Source: CAD feature listing. Evaluate the final solid. Frame: model axes, mm. Give positions to 0.01 mm unless a question says otherwise; leave off trailing zeros. Order: outer loops, then holes, each group sorted by start corner. A loop starts at its lowest first (then second) coordinate and runs counter-clockwise, first axis right, second up.
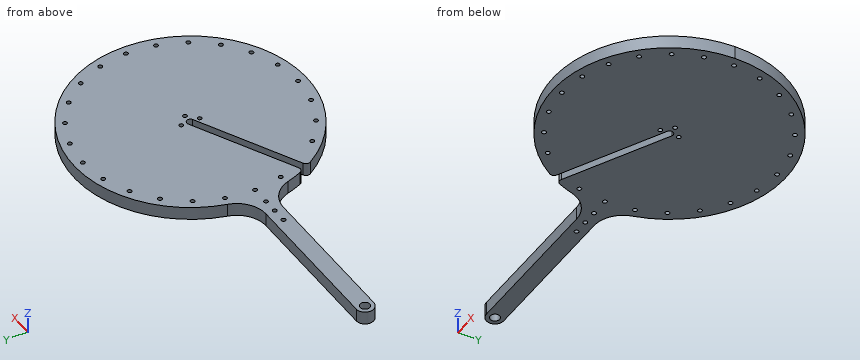
```python
from build123d import *

# Parameters (mm, degrees)
SKETCH1_R           = 1.4225
SKETCH1_R_2         = 1.450000001
SKETCH1_R_3         = 3.250000001
SKETCH1_R_4         = 1.45
BOSS_EXTRUDE2_DEPTH = 9
FILLET1_R           = 3
FILLET2_R           = 3


with BuildPart() as part:
    # Sketch1 → Boss-Extrude2 (new body)
    with BuildSketch(Plane.XY):
        with BuildLine():
            Line((-155.352886895, 10.211716756), (-51.913748531, 10.211716756))
            ThreePointArc((-51.913748531, 10.211716756), (-39.74822347, 6.086224622), (-32.601576204, -4.588283244))
            ThreePointArc((-32.601576204, -4.588283244), (-30.459614432, -11.337865429), (-27.729181359, -17.871592937))
            Line((-27.729181359, -17.871592937), (43.5118499, 18.439086832))
            ThreePointArc((43.5118499, 18.439086832), (46.874483182, 17.346979962), (45.782376313, 13.98434668))
            Line((45.782376313, 13.98434668), (-25.458654946, -22.326333089))
            ThreePointArc((-25.458654946, -22.326333089), (63.046973792, -61.643566474), (124.587919611, 13.13479368))
            ThreePointArc((124.587919611, 13.13479368), (56.661218885, 95.304455124), (-32.601576204, 37.011716756))
            ThreePointArc((-32.601576204, 37.011716756), (-39.74822347, 26.33720889), (-51.913748531, 22.211716756))
            Line((-51.913748531, 22.211716756), (-155.352886895, 22.211716756))
            ThreePointArc((-155.352886895, 22.211716756), (-161.352886895, 16.211716756), (-155.352886895, 10.211716756))
        make_face()
        with Locations((44.647113106, 22.561716756)):
            Circle(SKETCH1_R, mode=Mode.SUBTRACT)
        with Locations((-26.831398039, -2.940892579)):
            Circle(SKETCH1_R_2, mode=Mode.SUBTRACT)
        with Locations((-155.352886895, 16.211716756)):
            Circle(SKETCH1_R_3, mode=Mode.SUBTRACT)
        with Locations((-26.831398039, 35.364326096)):
            Circle(SKETCH1_R_2, mode=Mode.SUBTRACT)
        with Locations((-19.438766774, 53.211716759)):
            Circle(SKETCH1_R_2, mode=Mode.SUBTRACT)
        with Locations((-29.352886893, 16.211716758)):
            Circle(SKETCH1_R_2, mode=Mode.SUBTRACT)
        with Locations((-51.913748531, 16.211716758)):
            Circle(SKETCH1_R_4, mode=Mode.SUBTRACT)
        with Locations((-41.913748531, 16.211716758)):
            Circle(SKETCH1_R_4, mode=Mode.SUBTRACT)
        with Locations((-61.913748531, 16.211716758)):
            Circle(SKETCH1_R_4, mode=Mode.SUBTRACT)
        with Locations((50.997113106, 16.211716756)):
            Circle(SKETCH1_R, mode=Mode.SUBTRACT)
        with Locations((44.647113106, 9.861716756)):
            Circle(SKETCH1_R, mode=Mode.SUBTRACT)
        with Locations((116.125624253, -2.940892579)):
            Circle(SKETCH1_R_2, mode=Mode.SUBTRACT)
        with Locations((108.732992988, -20.788283242)):
            Circle(SKETCH1_R_2, mode=Mode.SUBTRACT)
        with Locations((96.973014915, -36.114185049)):
            Circle(SKETCH1_R_2, mode=Mode.SUBTRACT)
        with Locations((81.647113106, -47.874163121)):
            Circle(SKETCH1_R_2, mode=Mode.SUBTRACT)
        with Locations((63.799722443, -55.266794386)):
            Circle(SKETCH1_R_2, mode=Mode.SUBTRACT)
        with Locations((44.647113106, -57.788283242)):
            Circle(SKETCH1_R_2, mode=Mode.SUBTRACT)
        with Locations((25.494503768, -55.266794386)):
            Circle(SKETCH1_R_2, mode=Mode.SUBTRACT)
        with Locations((7.647113108, -47.874163121)):
            Circle(SKETCH1_R_2, mode=Mode.SUBTRACT)
        with Locations((-7.678788702, -36.114185049)):
            Circle(SKETCH1_R_2, mode=Mode.SUBTRACT)
        with Locations((-7.678788702, 68.537618566)):
            Circle(SKETCH1_R_2, mode=Mode.SUBTRACT)
        with Locations((7.647113108, 80.297596638)):
            Circle(SKETCH1_R_2, mode=Mode.SUBTRACT)
        with Locations((25.494503768, 87.690227903)):
            Circle(SKETCH1_R_2, mode=Mode.SUBTRACT)
        with Locations((44.647113106, 90.211716759)):
            Circle(SKETCH1_R_2, mode=Mode.SUBTRACT)
        with Locations((63.799722443, 87.690227903)):
            Circle(SKETCH1_R_2, mode=Mode.SUBTRACT)
        with Locations((81.647113106, 80.297596638)):
            Circle(SKETCH1_R_2, mode=Mode.SUBTRACT)
        with Locations((96.973014915, 68.537618566)):
            Circle(SKETCH1_R_2, mode=Mode.SUBTRACT)
        with Locations((108.732992988, 53.211716759)):
            Circle(SKETCH1_R_2, mode=Mode.SUBTRACT)
        with Locations((116.125624253, 35.364326096)):
            Circle(SKETCH1_R_2, mode=Mode.SUBTRACT)
        with Locations((118.647113104, 16.211716758)):
            Circle(SKETCH1_R_2, mode=Mode.SUBTRACT)
    extrude(amount=BOSS_EXTRUDE2_DEPTH)

    # Fillet1
    fillet1_edges = [part.edges().sort_by_distance(p)[0] for p in [
        (-27.729181359, -17.871592937, 4.5),
    ]]
    fillet(fillet1_edges, radius=FILLET1_R)

    # Fillet2
    fillet2_edges = [part.edges().sort_by_distance(p)[0] for p in [
        (-25.458654946, -22.326333089, 4.5),
    ]]
    fillet(fillet2_edges, radius=FILLET2_R)


solid = part.part
```
1) Section query C-C, the plane z = 1.5. Count the separate pieces of the cut face and the enclosed holes in it, and give its area (3 significant figures).
Report:
separate pieces: 1
enclosed holes: 30
area: 21,100 mm2
2) Section query B-B, the plane x = -97. Return the cut outline in (y, z).
Report:
outline: (10.21, 0) - (22.21, 0) - (22.21, 9) - (10.21, 9) - close
3) Section query D-D, the plane x = 89. Return the cut outline in (y, z), and give its area (3 significant figures).
Report:
outline: (-50.37, 0) - (82.79, 0) - (82.79, 9) - (-50.37, 9) - close
area: 1,200 mm2
4) Material intervals for L1, parallel to Y at x = 0, z = 7; L2, parallel to Y at x = -67.5, z = 8; L3, parallel to Y at x = 1, z = 6, sorted ascending.
Report:
L1: y = -50.17 to -9.35, -3.74 to 82.59
L2: y = 10.21 to 22.21
L3: y = -50.83 to -8.84, -3.23 to 83.26
5) Section query A-A, the plane x = -14. Return the cut outline in (y, z).
Report:
outline: (-38.2, 0) - (-16.49, 0) - (-16.49, 9) - (-38.2, 9) - close; (-10.87, 0) - (70.62, 0) - (70.62, 9) - (-10.87, 9) - close
6) Pin query (flat end, axial travel): pin 1 (3 mm diameter, centred on x = 87, z = 5.5, fed in from -Y); pin 2 (1 mm diameter, centred on y = 57.5, z = 8, fed in from +X); pin 3 (5 mm diameter, centred on y = 49, z = 1.5, fed in from +X). Return the tip coordinate at first contact, or that it passes through.
Report:
pin 1: stops at y = -52.57
pin 2: stops at x = 113.47
pin 3: stops at x = 118.69
